Can you work these out from the model? Positions are in its coordinate system, mm. Coordinates: 2 decimals unless noted, no trailing zeros. Order: outer loops, then holes, each group sorted by start corner. A loop starts at its lowest first (then second) coordinate and runs counter-clockwise, first axis right, second up. Notation, with made-up numbers: (83.5, 60) -> (132.5, 60) arc R25 cw to (132.5, 83) -> close; hole circle Ø11 at (49, -30). An arc over 180 degrees is marked (long way). Answer as a JSON object with one key per item and string values. Group by question number.
(1) I want a section at C-C, the plane z = 2.55. List the corners of the cut face in (x, y) for me, plus the area to 3 significant figures.
(2) For pin 1 (5.5 mm diameter, centred on x = 24, y = 24, fed in from +Z); pin 2 (4 mm diameter, centred on x = -24, y = -24, fed in from +Z); pin 3 (4.5 mm diameter, centred on x = -24, y = 24, fed in from +Z), each with a flat end and sliding along its axis, tell me the tip position at first contact or that it passes through.
(3) I need wall thicknesses on line 1 (X direction, y = 24, z = 0.3); line 2 (Y direction, x = -21.5, z = 2.8). Which ranges of each line are inside material? Lowest first, please.
(4) I want a section at A-A, the plane y = -24. List the corners of the cut face in (x, z) for me.
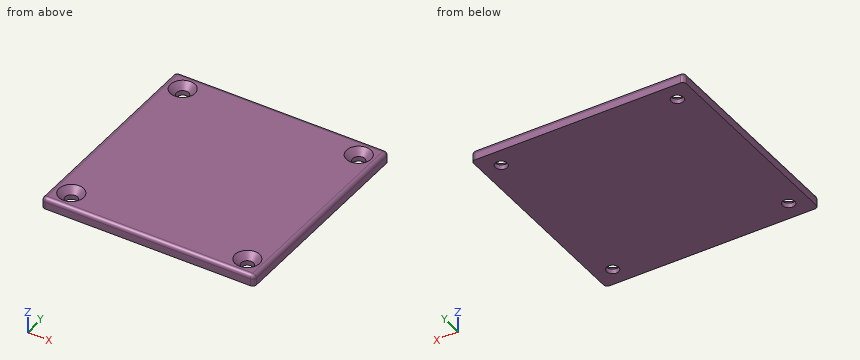
from build123d import *

# Parameters (mm, degrees)
F1_DEPTH       = 3
F2_R           = 1
F4_D           = 3.3
F4_CSINK_D     = 6.72
F4_CSINK_ANGLE = 90


with BuildPart() as f1:
    # F0 (on Top) → F1 (new body)
    with BuildSketch(Plane.XY):
        with BuildLine():
            Line((-28, -29), (28, -29))
            ThreePointArc((28, -29), (28.7071067812, -28.7071067812), (29, -28))
            Line((29, -28), (29, 28))
            ThreePointArc((29, 28), (28.7071067812, 28.7071067812), (28, 29))
            Line((28, 29), (-28, 29))
            ThreePointArc((-28, 29), (-28.7071067812, 28.7071067812), (-29, 28))
            Line((-29, 28), (-29, -28))
            ThreePointArc((-29, -28), (-28.7071067812, -28.7071067812), (-28, -29))
        make_face()
    extrude(amount=F1_DEPTH)

    # F2
    f2_edges = [f1.edges().sort_by_distance(p)[0] for p in [
        (29, 0, 3),
    ]]
    fillet(f2_edges, radius=F2_R)

    # F4 (through all)
    with Locations(Plane.XY.offset(3)):
        with Locations((-24, 24), (24, 24), (-24, -24), (24, -24)):
            CounterSinkHole(F4_D / 2, F4_CSINK_D / 2, counter_sink_angle=F4_CSINK_ANGLE)


solid = f1.part
Computed values:
{
 "1": {"outline": "(-28.84, -28) arc R0.84 ccw to (-28, -28.84) -> (28, -28.84) arc R0.84 ccw to (28.84, -28) -> (28.84, 28) arc R0.84 ccw to (28, 28.84) -> (-28, 28.84) arc R0.84 ccw to (-28.84, 28) -> close; hole circle Ø5.82 at (-24, -24); hole circle Ø5.82 at (-24, 24); hole circle Ø5.82 at (24, -24); hole circle Ø5.82 at (24, 24)", "area": "3,220 mm2"},
 "2": {"pin 1": "stops at z = 2.39", "pin 2": "stops at z = 1.64", "pin 3": "stops at z = 1.89"},
 "3": {"line 1": "x = -29 to -25.65, -22.35 to 22.35, 25.65 to 29", "line 2": "y = -28.6 to -25.93, -22.07 to 22.07, 25.93 to 28.6"},
 "4": {"outline": "(-29, 0) -> (-25.65, 0) -> (-25.65, 1.29) -> (-27.36, 3) -> (-28, 3) arc R1 ccw to (-29, 2) -> close; (-22.35, 0) -> (22.35, 0) -> (22.35, 1.29) -> (20.64, 3) -> (-20.64, 3) -> (-22.35, 1.29) -> close; (25.65, 0) -> (29, 0) -> (29, 2) arc R1 ccw to (28, 3) -> (27.36, 3) -> (25.65, 1.29) -> close"}
}
